```python
from build123d import *

# Parameters (mm, degrees)
F0_R     = 40
F0_R_2   = 0.75
F1_DEPTH = 2


with BuildPart() as f1:
    # F0 (on Top) → F1 (new body)
    with BuildSketch(Plane.XY):
        Circle(F0_R)
        with Locations((-20.78299, -25.164945)):
            Circle(F0_R_2, mode=Mode.SUBTRACT)
        with Locations((-26.792528, -20.156994)):
            Circle(F0_R_2, mode=Mode.SUBTRACT)
        with Locations((-10.516693, -31.174485)):
            Circle(F0_R_2, mode=Mode.SUBTRACT)
        with Locations((-13.521464, -21.409065)):
            Circle(F0_R_2, mode=Mode.SUBTRACT)
        with Locations((-2.00318, -25.415344)):
            Circle(F0_R_2, mode=Mode.SUBTRACT)
        with Locations((-31.049285, -14.147457)):
            Circle(F0_R_2, mode=Mode.SUBTRACT)
        with Locations((-20.532593, -14.647896)):
            Circle(F0_R_2, mode=Mode.SUBTRACT)
        with Locations((-32.050874, -6.385135)):
            Circle(F0_R_2, mode=Mode.SUBTRACT)
        with Locations((-24.789348, -5.633006)):
            Circle(F0_R_2, mode=Mode.SUBTRACT)
        with Locations((-13.085132, -10.563891)):
            Circle(F0_R_2, mode=Mode.SUBTRACT)
        with Locations((-8.170747, -15.973391)):
            Circle(F0_R_2, mode=Mode.SUBTRACT)
        with Locations((-1.00159, -18.153816)):
            Circle(F0_R_2, mode=Mode.SUBTRACT)
        with Locations((-1.00159, -10.641892)):
            Circle(F0_R_2, mode=Mode.SUBTRACT)
        with Locations((-17.265331, -2.690971)):
            Circle(F0_R_2, mode=Mode.SUBTRACT)
        with Locations((-8.823515, -7.313374)):
            Circle(F0_R_2, mode=Mode.SUBTRACT)
        with Locations((0, -32.5)):
            Circle(F0_R_2, mode=Mode.SUBTRACT)
        with Locations((12.019077, -30.17354)):
            Circle(F0_R_2, mode=Mode.SUBTRACT)
        with Locations((5.001707, -25.1524)):
            Circle(F0_R_2, mode=Mode.SUBTRACT)
        with Locations((11.018466, -22.407565)):
            Circle(F0_R_2, mode=Mode.SUBTRACT)
        with Locations((20.031797, -25.415681)):
            Circle(F0_R_2, mode=Mode.SUBTRACT)
        with Locations((26.041336, -20.156994)):
            Circle(F0_R_2, mode=Mode.SUBTRACT)
        with Locations((6.498813, -16.62863)):
            Circle(F0_R_2, mode=Mode.SUBTRACT)
        with Locations((18.033735, -17.151887)):
            Circle(F0_R_2, mode=Mode.SUBTRACT)
        with Locations((12.0117, -11.374607)):
            Circle(F0_R_2, mode=Mode.SUBTRACT)
        with Locations((5.428696, -8.52426)):
            Circle(F0_R_2, mode=Mode.SUBTRACT)
        with Locations((9.956572, -2.640874)):
            Circle(F0_R_2, mode=Mode.SUBTRACT)
        with Locations((15.014591, -4.10834)):
            Circle(F0_R_2, mode=Mode.SUBTRACT)
        with Locations((20.036818, -13.646242)):
            Circle(F0_R_2, mode=Mode.SUBTRACT)
        with Locations((24.291573, -1.626389)):
            Circle(F0_R_2, mode=Mode.SUBTRACT)
        with Locations((30.298091, -9.640303)):
            Circle(F0_R_2, mode=Mode.SUBTRACT)
        with Locations((32.050874, -1.627584)):
            Circle(F0_R_2, mode=Mode.SUBTRACT)
        with Locations((-32.050874, 2.378776)):
            Circle(F0_R_2, mode=Mode.SUBTRACT)
        with Locations((-24.538951, 3.381884)):
            Circle(F0_R_2, mode=Mode.SUBTRACT)
        with Locations((-31.049285, 10.89229)):
            Circle(F0_R_2, mode=Mode.SUBTRACT)
        with Locations((-22.535771, 12.396773)):
            Circle(F0_R_2, mode=Mode.SUBTRACT)
        with Locations((-28.044516, 17.402625)):
            Circle(F0_R_2, mode=Mode.SUBTRACT)
        with Locations((-16.12178, 5.494459)):
            Circle(F0_R_2, mode=Mode.SUBTRACT)
        with Locations((-14.562273, 9.657283)):
            Circle(F0_R_2, mode=Mode.SUBTRACT)
        with Locations((-8.088846, 4.472589)):
            Circle(F0_R_2, mode=Mode.SUBTRACT)
        with Locations((-1.752782, 8.638713)):
            Circle(F0_R_2, mode=Mode.SUBTRACT)
        with Locations((-18.028617, 17.65546)):
            Circle(F0_R_2, mode=Mode.SUBTRACT)
        with Locations((-8.559517, 15.310555)):
            Circle(F0_R_2, mode=Mode.SUBTRACT)
        with Locations((-1.752782, 15.649842)):
            Circle(F0_R_2, mode=Mode.SUBTRACT)
        with Locations((-21.784579, 24.413751)):
            Circle(F0_R_2, mode=Mode.SUBTRACT)
        with Locations((-12.019078, 21.662077)):
            Circle(F0_R_2, mode=Mode.SUBTRACT)
        with Locations((-15.023848, 28.420113)):
            Circle(F0_R_2, mode=Mode.SUBTRACT)
        with Locations((-0.500794, 24.413751)):
            Circle(F0_R_2, mode=Mode.SUBTRACT)
        with Locations((-8.012719, 30.673688)):
            Circle(F0_R_2, mode=Mode.SUBTRACT)
        with Locations((-0.751193, 32.676868)):
            Circle(F0_R_2, mode=Mode.SUBTRACT)
        with Locations((0.083299, 0.782396)):
            Circle(F0_R_2, mode=Mode.SUBTRACT)
        with Locations((8.358954, 3.596777)):
            Circle(F0_R_2, mode=Mode.SUBTRACT)
        with Locations((16.523292, 5.051284)):
            Circle(F0_R_2, mode=Mode.SUBTRACT)
        with Locations((7.431873, 16.293498)):
            Circle(F0_R_2, mode=Mode.SUBTRACT)
        with Locations((13.338599, 10.725901)):
            Circle(F0_R_2, mode=Mode.SUBTRACT)
        with Locations((15.27423, 17.655458)):
            Circle(F0_R_2, mode=Mode.SUBTRACT)
        with Locations((24.040258, 5.635606)):
            Circle(F0_R_2, mode=Mode.SUBTRACT)
        with Locations((30.047698, 9.389905)):
            Circle(F0_R_2, mode=Mode.SUBTRACT)
        with Locations((21.535313, 11.895946)):
            Circle(F0_R_2, mode=Mode.SUBTRACT)
        with Locations((26.291735, 18.905008)):
            Circle(F0_R_2, mode=Mode.SUBTRACT)
        with Locations((4.00636, 23.414971)):
            Circle(F0_R_2, mode=Mode.SUBTRACT)
        with Locations((14.022258, 27.418524)):
            Circle(F0_R_2, mode=Mode.SUBTRACT)
        with Locations((7.511923, 30.924087)):
            Circle(F0_R_2, mode=Mode.SUBTRACT)
        with Locations((20.031797, 24.413751)):
            Circle(F0_R_2, mode=Mode.SUBTRACT)
    extrude(amount=F1_DEPTH)


solid = f1.part
```
Could you check a few things on this model? Use its own coordinates, in mm. Round coordinates to 2 decimals unless told otherwise and drop trailing zeros. Put each result on its own line as item: value.
Q1. Please list where these lines run through material, in increasing order: line 1 (Y direction, x = 5, z = 1.5); line 2 (X direction, y = -14.5, z = 1.7); line 3 (Y direction, x = -25, z = 0.2). Write a range as from..to.
Checks:
line 1: -39.69..-25.9, -24.4..-9.14, -7.91..39.69
line 2: -37.28..-31.71, -30.39..-21.27, -19.8..37.28
line 3: -31.22..-6.35, -4.91..2.79, 3.97..31.22
Q2. For pin 1 Ø2 at (x, y) = (-10.52, -31.17) entering from -Z; pin 2 Ø1 at (y, z) = (-11, 1) entering from -X, each with a flat end and sliding along its axis, tell me the tip position at first contact or that it passes through.
Checks:
pin 1: z = 0
pin 2: x = -38.6
Q3. I want a section at A-A on z = 0.75. Give the number of separate pieces and of enclosed holes in the cut face, and give its area (3 significant figures).
Checks:
separate pieces: 1
enclosed holes: 63
area: 4,920 mm2
